Model file for the job. Use its own axes, mm. Face numbers are marked on the shaded views. A direction names the side the tool comes from. Give positions to 0.01 mm unless a question says otherwise; leave off trailing zeros. Write each loop counter-clockwise with the first axis right and the second up, starting at its lowest first coordinate (ties: lowest second). Pieces come first, ordered by that corner, then holes. Notation, with made-up numbers: (71.5, 89) - (79.5, 89) arc R31 ccw to (79.5, 115) - close; hole circle Ø1 at (82, -24.5). An arc over 180 degrees is marked (long way). One line per item, written item: value. Start each with the question number.
(1) Drop flat-ended pins along their axis: P1, Ø8, axis at x = 3.5, y = 34.5, coming from the -Z side; P2, Ø6, axis at y = 25, z = 26.5, coming from the +X side; P3, Ø6, axis at x = 6.5, z = 80.5, coming from the +Y side; P4, Ø3, axis at x = 7.5, y = 8.5, coming from the +Z side. Give the stop position or say it passes through.
(2) 3-axis set-ups, long thin cutter, end or side, ignore diameter. For the marked faces 1, 2 and 3: which of +Z, -Z, +X, -X, +Y, -Y reach the whole face in a straight line?
(3) Cut at C-C, the plane y = 4. List the corners of the cut face in (x, z).
(4) Probe L1, parallel to X at y = 1.25, z = 99.5; L2, parallel to Y at x = 10, z = 9.85; L3, parallel to Y at x = 10, z = 3. List the from-to ranges inside material, lowest first.
(5) Cut at D-D, the plane x = 9. List the corners of the cut face in (y, z).
(6) Cut at A-A, the plane y = 30. List the corners of the cut face in (x, z).
(7) Cut at B-B, the plane z = 99.5. List the corners of the cut face in (x, y).
from build123d import *

# Parameters (mm, degrees)
SKETCH3_W                = 20
SKETCH3_H                = 107.5
SKETCH3_R                = 6.15
BOSS_EXTRUDE2_DEPTH      = 5
BOSS_EXTRUDE3_DEPTH      = 4
BOSS_EXTRUDE3_DEPTH_BACK = 4
SKETCH5_R                = 2.65
CUT_EXTRUDE1_DEPTH       = 12
SKETCH6_W                = 4
SKETCH6_H                = 8
CUT_EXTRUDE2_DEPTH       = 121.451234946
FILLET1_R                = 3


with BuildPart() as part:
    # Sketch3 → Boss-Extrude2 (new body)
    with BuildSketch(Plane(origin=(0, 0, 0), x_dir=(1, 0, 0), z_dir=(0, 1, 0))):
        with Locations((10, -53.75)):
            Rectangle(SKETCH3_W, SKETCH3_H)
        with Locations(Location((10, -99.5, 0), (0, 0, 270))):
            Circle(SKETCH3_R, mode=Mode.SUBTRACT)
    extrude(amount=BOSS_EXTRUDE2_DEPTH)

    # Sketch4 → Boss-Extrude3 (add, two sides: drawn at the far end of the back side and taken through both)
    with BuildSketch(Plane(origin=(10, 0, 0), x_dir=(0, 0, -1), z_dir=(1, 0, 0)).offset(-BOSS_EXTRUDE3_DEPTH_BACK)):
        Polygon((0, 5), (0, 52.5), (-47.5, 5), align=None)
    extrude(amount=BOSS_EXTRUDE3_DEPTH + BOSS_EXTRUDE3_DEPTH_BACK)

    # Sketch5 → Cut-Extrude1 (cut)
    with BuildSketch(Plane(origin=(0, 0, 0), x_dir=(-1, 0, 0), z_dir=(0, 0, -1))):
        with Locations((-10, 30)):
            Circle(SKETCH5_R)
    extrude(amount=-CUT_EXTRUDE1_DEPTH, mode=Mode.SUBTRACT)

    # Sketch6 → Cut-Extrude2 (cut, through all)
    with BuildSketch(Plane(origin=(14, 0, 0), x_dir=(0, 0, -1), z_dir=(1, 0, 0))):
        with Locations((-7, 30)):
            Rectangle(SKETCH6_W, SKETCH6_H)
    extrude(amount=-CUT_EXTRUDE2_DEPTH, mode=Mode.SUBTRACT)

    # Fillet1
    fillet1_edges = [part.edges().sort_by_distance(p)[0] for p in [
        (20, 2.5, 107.5),
        (0, 2.5, 107.5),
        (6, 5, 23.75),
        (10, 5, 47.5),
        (14, 5, 23.75),
        (10, 52.5, 0),
        (20, 2.5, 0),
        (0, 2.5, 0),
    ]]
    fillet(fillet1_edges, radius=FILLET1_R - 0.0001)  # a hair under: the kernel refuses the full size


solid = part.part
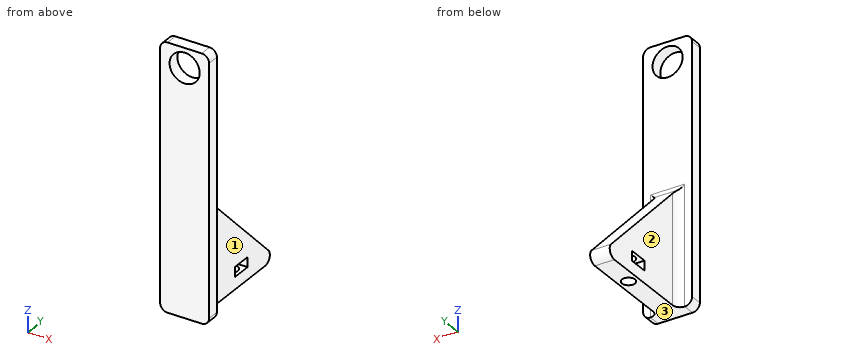
Answers follow:
1. P1: stops at z = 0
1. P2: stops at x = 14
1. P3: stops at y = 5
1. P4: stops at z = 45.5
2. face 1: +Z, -Z, +X, +Y
2. face 2: +Z, -Z, -X, +Y
2. face 3: -Z, +X, -X, +Y, -Y
3. outline: (0, 3) arc R3 ccw to (3, 0) - (17, 0) arc R3 ccw to (20, 3) - (20, 104.5) arc R3 ccw to (17, 107.5) - (3, 107.5) arc R3 ccw to (0, 104.5) - close; hole circle Ø12.3 at (10, 99.5)
4. L1: x = 0 to 3.85, 16.15 to 20
4. L2: y = 0 to 27.35, 32.65 to 42.65
4. L3: y = 0 to 27.35, 32.65 to 48.26
5. outline: (0, 0) - (27.55, 0) - (27.55, 5) - (26, 5) - (26, 9) - (27.55, 9) - (27.55, 12) - (32.45, 12) - (32.45, 9) - (34, 9) - (34, 5) - (32.45, 5) - (32.45, 0) - (45.26, 0) arc R3 ccw to (47.38, 5.12) - (5.88, 46.62) arc R3 cw to (5, 48.74) - (5, 93.43) - (0, 93.43) - close; (0, 105.57) - (5, 105.57) - (5, 107.5) - (0, 107.5) - close
6. outline: (6, 0) - (7.35, 0) - (7.35, 5) - (6, 5) - close; (6, 9) - (7.35, 9) - (7.35, 12) - (12.65, 12) - (12.65, 9) - (14, 9) - (14, 22.5) - (6, 22.5) - close; (12.65, 0) - (14, 0) - (14, 5) - (12.65, 5) - close
7. outline: (0, 0) - (3.85, 0) - (3.85, 5) - (0, 5) - close; (16.15, 0) - (20, 0) - (20, 5) - (16.15, 5) - close
